For this review, take the finished solid that the model builds, in its own axes (mm). Face numbers are marked on the shaded views. A direction names the side the tool comes from. Round coordinates to 2 decimals unless told otherwise and drop trailing zeros. Write each loop counter-clockwise with the first axis right and the second up, starting at its lowest first coordinate (ties: lowest second). Pieces come first, ordered by that corner, then holes. Notation, with made-up numbers: M 15.25,-8.75 L 23.25,-8.75 A28 cw 23.25,27.25 Z; hole C 64.25,55.25 d11. An arc over 180 degrees is marked long. Use one line per item in the form item = value. Start each with the question number.
Item 1: Add section B-B (x = -121). State the section outline as (y, z) points.
Item 2: Add section A-A (z = 107.5). State the section outline as (x, y) points.
Item 3: For the marked faces 1 and 2, list the 3-axis set-ups (+Z, -Z, +X, -X, +Y, -Y) from which the entire face can be reached by the end or side of a thin tool; tool diameter is ignored.
Item 4: Add section D-D (z = 37.5). State the section outline as (x, y) points, and give its area (3 significant figures).
Item 5: Add section C-C (y = -5.5). State the section outline as (x, z) points.
Item 6: For line 1 (X direction, y = -78.5, z = 41.5); line 2 (Y direction, x = -110, z = 91.5), list the stretches that pass through material, from the lowest coordinate up. Write a range as [from, to].
Item 7: For P1, Ø1.5, axis at x = -57, z = 116, coming from the -Y side; P2, Ø2.5, axis at x = -79, y = 1.5, coming from the -Z side; P3, Ø0.9, axis at y = 1, z = 27.5, coming from the +X side, all flat-tipped, find the tip position at first contact; note any pin that passes through.
Autodesk Inventor part; units mm, degrees
ref_plane "YZ Plane" through (0, 0, 0) normal (1, 0, 0) x (0, 1, 0)
ref_plane "XZ Plane" through (0, 0, 0) normal (0, 1, 0) x (-1, 0, 0)
ref_plane "XY Plane" through (0, 0, 0) normal (0, 0, 1) x (1, 0, 0)
sketch "Sketch1" plane through (0, 0, 0) normal (0, 1, 0) x (-1, 0, 0)
  line L0 (110, -80) -> (-110, -80)
  line L1 (-110, -80) -> (-110, 80)
  line L2 (-110, 80) -> (110, 80)
  line L3 (110, 80) -> (110, -80)
  line L4 (320.2117, -53.5522) -> (168.036, -53.5522) construction
  line L5 (168.036, -53.5522) -> (168.036, 90.1689) construction
  line L6 (168.036, 90.1689) -> (320.2117, 90.1689) construction
  line L7 (320.2117, 90.1689) -> (320.2117, -53.5522) construction
  line L8 (124.3, -89.75) -> (-124.3, -89.75) construction
  line L9 (-124.3, -89.75) -> (-124.3, 89.75) construction
  line L10 (-124.3, 89.75) -> (124.3, 89.75) construction
  line L11 (124.3, 89.75) -> (124.3, -89.75) construction
  line L12 (124.3, -89.75) -> (-124.3, 89.75) construction
  line L13 (-124.3, -89.75) -> (124.3, 89.75) construction
  line L14 (-152.4, -107.95) -> (152.4, -107.95)
  line L15 (152.4, -107.95) -> (152.4, 107.95)
  line L16 (152.4, 107.95) -> (-152.4, 107.95)
  line L17 (-152.4, 107.95) -> (-152.4, -107.95)
  line L18 (-152.4, -107.95) -> (152.4, 107.95) construction
  line L19 (152.4, -107.95) -> (-152.4, 107.95) construction
  line L20 (177.8, 133.35) -> (177.8, -133.35)
  line L21 (177.8, -133.35) -> (-177.8, -133.35)
  line L22 (-177.8, -133.35) -> (-177.8, 133.35)
  line L23 (-177.8, 133.35) -> (177.8, 133.35)
  point P0 (0, 0)
  dimension "d11" = 220
  dimension "d12" = 160
  dimension "d15" = 248.6
  dimension "d16" = 179.5
  dimension "d18" = 304.8
  dimension "d19" = 215.9
  dimension "d22" = 25.4
extrude "Top" add sketch "Sketch1" along normal blind 25.4 contours L17 L16 L15 L14 | L20 L21 L22 L23
sketch "Sketch3" plane through (177.8, 0, 133.35) normal (1, 0, 0) x (0, 0, -1)
  line L0 (0, 0) -> (0, 25.4)
  line L1 (266.7, 0) -> (266.7, 25.4)
  line L2 (0, 0) -> (266.7, 0)
  line L3 (266.7, 0) -> (266.7, -266.7)
  line L4 (266.7, -266.7) -> (0, -266.7)
  line L5 (0, -266.7) -> (0, 0)
  point P0 (133.35, 0)
  dimension "d25" = 266.7
extrude "Right" add sketch "Sketch3" against normal blind 50.8
sketch "Sketch4" plane through (-177.8, 0, -133.35) normal (-1, 0, 0) x (0, 0, 1)
  line L0 (0, 0) -> (0, 25.4)
  line L1 (266.7, -266.7) -> (266.7, 0)
  line L2 (0, 0) -> (266.7, 0)
  line L3 (266.7, 0) -> (266.7, -266.7)
  line L4 (266.7, -266.7) -> (0, -266.7)
  line L5 (0, -266.7) -> (0, 0)
  point P0 (133.35, 0)
  dimension "d28" = 266.7
extrude "Left" add sketch "Sketch4" against normal blind 50.8
sketch "Sketch5" plane through (0, 0, 0) normal (1, 0, 0) x (0, 1, 0)
  line L0 (-266.7, -133.35) -> (25.4, -133.35)
  line L1 (-266.7, 133.35) -> (-266.7, -133.35)
  line L2 (0, -133.35) -> (-266.7, 133.35)
  line L3 (-266.7, 133.35) -> (-275.6803, 124.3697)
  line L4 (-275.6803, 124.3697) -> (-8.9803, -142.3303)
  line L5 (-8.9803, -142.3303) -> (0, -133.35)
  point P0 (0, 0)
  dimension "d31" = 12.7
extrude "Plexiglass Cut" cut sketch "Sketch5" along normal mid plane 304.8 contours L4 L1 L2 L0 | L0 L5 L4 | L4 L3 L1
sketch "Sketch6" plane through (-177.8, -266.7, -133.35) normal (0, -1, 0) x (1, 0, 0)
  line L0 (0, 0) -> (0, 266.7)
  line L1 (355.6, 0) -> (0, 0)
  line L2 (0, 266.7) -> (355.6, 266.7)
  line L3 (355.6, 266.7) -> (355.6, 0)
  line L4 (355.6, 0) -> (0, 0)
  line L5 (0, 0) -> (0, 266.7)
  point P0 (177.8, 133.35)
extrude "Bottom" add sketch "Sketch6" along normal blind 25.4
sketch "Sketch9" plane through (0, 25.4, 0) normal (0, 1, 0) x (1, 0, 0)
  line L0 (177.8, -133.35) -> (127, -133.35)
  line L1 (177.8, 133.35) -> (-177.8, 133.35)
  line L2 (177.8, -133.35) -> (-177.8, -133.35)
  line L3 (-177.8, -133.35) -> (-177.8, 133.35)
  line L4 (-177.8, 133.35) -> (177.8, 133.35)
  line L5 (177.8, 133.35) -> (177.8, -133.35)
  point P0 (0, 0)
extrude "Top Flattening" cut sketch "Sketch9" against normal blind 22.4
sketch "Sketch10" plane through (0, 3, 0) normal (0, 1, 0) x (1, 0, 0)
  line L0 (-177.8, -133.35) -> (-177.8, 133.35)
  line L1 (-155.4106, 133.35) -> (-177.8, 133.35)
  line L2 (-177.8, 133.35) -> (-177.8, -133.35)
  line L3 (-177.8, -133.35) -> (-155.4106, -133.35)
  line L4 (-155.4106, -133.35) -> (-155.4106, 133.35)
  line L5 (177.8, 133.35) -> (177.8, -133.35)
  line L6 (177.8, -133.35) -> (155.4106, -133.35)
  line L7 (155.4106, -133.35) -> (155.4106, 133.35)
  line L8 (155.4106, 133.35) -> (177.8, 133.35)
  line L9 (152.4, -115.3895) -> (152.4, 133.35)
  point P0 (0, 0)
  point P1 (-177.8, 0)
  dimension "d48" = 22.3894
  dimension "d49" = 22.3894
extrude "Outer Side Flattening" cut sketch "Sketch10" against normal through all
sketch "Sketch11" plane through (-177.8, -292.1, -133.35) normal (0, -1, 0) x (1, 0, 0)
  line L0 (22.3894, 0) -> (333.2106, 0)
  line L1 (333.2106, 0) -> (22.3894, 0)
  line L2 (22.3894, 0) -> (22.3894, 266.7)
  line L3 (22.3894, 266.7) -> (333.2106, 266.7)
  line L4 (333.2106, 266.7) -> (333.2106, 0)
  point P0 (177.8, 133.35)
extrude "Bottom Flattening" cut sketch "Sketch11" against normal blind 22.4
sketch "Sketch12" plane through (155.4106, 3, -133.35) normal (0, 0, -1) x (-1, 0, 0)
  line L0 (155.4106, -3) -> (155.4106, -269.7) construction
  line L1 (7.0106, -269.7) -> (7.0106, -3)
  line L2 (7.0106, -3) -> (303.8106, -3)
  line L3 (303.8106, -3) -> (303.8106, -269.7)
  line L4 (303.8106, -269.7) -> (7.0106, -269.7)
  line L5 (7.0106, -269.7) -> (303.8106, -3) construction
  line L6 (7.0106, -3) -> (303.8106, -269.7) construction
  point P0 (155.4106, -136.35)
  point P1 (155.4106, -3)
  dimension "d54" = 296.8
extrude "Inner Flattening" cut sketch "Sketch12" against normal through all
sketch "Sketch13" plane through (-155.4106, 3, 133.35) normal (0, 0, 1) x (1, 0, 0)
  line L0 (310.8211, -272.7) -> (310.8211, 0)
  line L1 (0, -272.7) -> (310.8211, -272.7)
  line L2 (310.8211, -136.35) -> (0, -136.35)
  line L3 (0, -136.35) -> (0, -272.7)
  line L4 (0, -272.7) -> (310.8211, -272.7)
  line L5 (310.8211, -272.7) -> (310.8211, -136.35)
  point P0 (155.4106, -3)
extrude "Bottom Cut" cut sketch "Sketch13" against normal through all
sketch "Sketch14" plane through (0, 3, 0) normal (0, 1, 0) x (1, 0, 0)
  line L0 (-155.4106, -133.35) -> (-148.4, -133.35)
  line L1 (0, 0) -> (-155.4106, 0)
  line L2 (-155.4106, 0) -> (-155.4106, -133.35)
  line L3 (-155.4106, -133.35) -> (0, -133.35)
  line L4 (0, -133.35) -> (0, 0)
  line L5 (-155.4106, 133.35) -> (155.4106, 133.35)
  line L6 (-155.4106, -133.35) -> (155.4106, -133.35)
  line L7 (155.4106, -133.35) -> (155.4106, 133.35)
  line L8 (155.4106, 133.35) -> (-155.4106, 133.35)
  line L9 (-155.4106, 133.35) -> (-155.4106, -133.35)
extrude "Quarter Cut" cut sketch "Sketch14" against normal through all contours L9 L5 L7 L6 L4 L1
properties part number "Apple iPad 2022 Hologram"
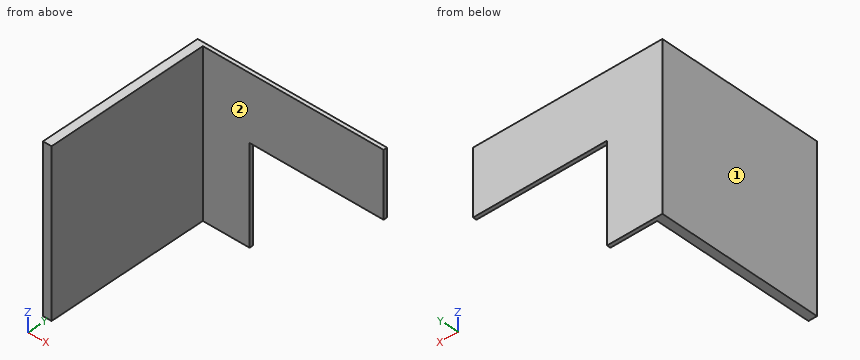
Calculated:
q1.outline = M 0,0 L 3,0 L 3,133.35 L 0,133.35 Z
q2.outline = M -155.41,-133.35 L -148.4,-133.35 L -148.4,0 L 0,0 L 0,3 L -155.41,3 Z
q3.face_1 = +Z, -Z, -X, +Y, -Y
q3.face_2 = +Z, -Z, +X, -Y
q4.outline = M -155.41,-133.35 L -148.4,-133.35 L -148.4,0 L -110,0 L -110,3 L -155.41,3 Z
q4.area = 1,070 mm^2
q5.outline = M -155.41,0 L -148.4,0 L -148.4,133.35 L -155.41,133.35 Z
q6.line_1 = [-155.41, -148.4]
q6.line_2 = [0, 3]
q7.P1 = 0
q7.P2 = 80
q7.P3 = -110
